Geometry check sheet. Reference: the model listing, model coordinates, mm. Round coordinates to 2 decimals unless told otherwise and drop trailing zeros. Loops run counter-clockwise (first coordinate to the right, second up) from the corner with the lowest first, then second, coordinate; pieces in that order, holes last. Notation, with made-up numbers: M -29,-33.5 L -7,-33.5 A21 ccw -7,-20.5 Z; hole C 18.5,55.5 d9. An arc over 180 degrees is marked long. Write item = value, one per line.
from build123d import *

# Parameters (mm, degrees)
F1_DEPTH = 3.048


with BuildPart() as f1:
    # F0 (on Front) → F1 (new body)
    with BuildSketch(Plane.XZ):
        with BuildLine():
            ThreePointArc((6.209856088, 64.9557709646), (6.2206928765, 65.1675907882), (6.224306538, 65.3796568513))
            ThreePointArc((6.224306538, 65.3796568513), (-2.0871396142, 71.2436009258), (-4.824583776, 61.4470517012))
            ThreePointArc((-4.824583776, 61.4470517012), (-2.6706040451, 59.7573916572), (0, 59.1553503133))
            ThreePointArc((0, 59.1553503133), (4.2487407654, 60.8310093834), (6.209856088, 64.9557709646))
        make_face()
        with BuildLine():
            ThreePointArc((0, 59.1553503133), (-2.6706040451, 59.7573916572), (-4.824583776, 61.4470517012))
            Line((-4.824583776, 61.4470517012), (-8.1232850213, 47.4475871287))
            ThreePointArc((-8.1232850213, 47.4475871287), (-5.1805872599, 52.0766598943), (0, 53.8792414952))
            Line((0, 53.8792414952), (0, 59.1553503133))
        make_face()
        with BuildLine():
            Line((7.9024256694, 48.2173679334), (6.209856088, 64.9557709646))
            ThreePointArc((6.209856088, 64.9557709646), (4.2487407654, 60.8310093834), (0, 59.1553503133))
            Line((0, 59.1553503133), (0, 53.8792414952))
            ThreePointArc((0, 53.8792414952), (4.8606878035, 52.3176828203), (7.9024256694, 48.2173679334))
        make_face()
        with BuildLine():
            ThreePointArc((0, 53.8792414952), (-5.1805872599, 52.0766598943), (-8.1232850213, 47.4475871287))
            ThreePointArc((-8.1232850213, 47.4475871287), (-6.5431667331, 40.3529059013), (0, 37.1877448272))
            Line((0, 37.1877448272), (0, 53.8792414952))
        make_face()
        with BuildLine():
            ThreePointArc((0, 37.1877448272), (-6.5431667331, 40.3529059013), (-8.1232850213, 47.4475871287))
            Line((-8.1232850213, 47.4475871287), (-8.9761791751, 43.8279621303))
            Line((-8.9761791751, 43.8279621303), (-7.522948678, 9.569606592))
            Line((-7.522948678, 9.569606592), (-5.7813609054, 9.6774364228))
            ThreePointArc((-5.7813609054, 9.6774364228), (-3.1997914593, 11.7007529388), (0, 12.4216171046))
            Line((0, 12.4216171046), (0, 37.1877448272))
        make_face()
        with BuildLine():
            Line((8.2797434874, 44.4859421904), (7.9024256694, 48.2173679334))
            ThreePointArc((7.9024256694, 48.2173679334), (4.8606878035, 52.3176828203), (0, 53.8792414952))
            Line((0, 53.8792414952), (0, 37.1877448272))
            ThreePointArc((0, 37.1877448272), (5.5185559019, 39.2727379343), (8.2797434874, 44.4859421904))
        make_face()
        with BuildLine():
            ThreePointArc((8.345748334, 45.5334931612), (8.2341718199, 46.893614367), (7.9024256694, 48.2173679334))
            Line((7.9024256694, 48.2173679334), (8.2797434874, 44.4859421904))
            ThreePointArc((8.2797434874, 44.4859421904), (8.3292307769, 45.0086789855), (8.345748334, 45.5334931612))
        make_face()
        with BuildLine():
            ThreePointArc((8.2797434874, 44.4859421904), (5.5185559019, 39.2727379343), (0, 37.1877448272))
            Line((0, 37.1877448272), (0, 12.4216171046))
            ThreePointArc((0, 12.4216171046), (5.2764963843, 10.2360207404), (7.4620927485, 4.9595243561))
            ThreePointArc((7.4620927485, 4.9595243561), (7.4592970858, 4.7552814289), (7.4509121924, 4.5511915405))
            Line((7.4509121924, 4.5511915405), (9.1615496203, 35.7654578984))
            Line((9.1615496203, 35.7654578984), (8.2797434874, 44.4859421904))
        make_face()
        with BuildLine():
            ThreePointArc((7.4620927485, 4.9595243561), (5.2764963843, 10.2360207404), (0, 12.4216171046))
            ThreePointArc((0, 12.4216171046), (-3.1997914593, 11.7007529388), (-5.7813609054, 9.6774364228))
            ThreePointArc((-5.7813609054, 9.6774364228), (-6.8181639984, 7.9919273436), (-7.3754788979, 6.0931641639))
            Line((-7.3754788979, 6.0931641639), (-7.2529785413, 3.2053492032))
            ThreePointArc((-7.2529785413, 3.2053492032), (-6.1468484582, 0.7287936603), (-4.2285927984, -1.1887950186))
            ThreePointArc((-4.2285927984, -1.1887950186), (3.2913062747, -1.737499699), (7.4509121924, 4.5511915405))
            ThreePointArc((7.4509121924, 4.5511915405), (7.4592970858, 4.7552814289), (7.4620927485, 4.9595243561))
        make_face()
        with BuildLine():
            Line((-5.7813609054, 9.6774364228), (-7.522948678, 9.569606592))
            Line((-7.522948678, 9.569606592), (-7.3754788979, 6.0931641639))
            ThreePointArc((-7.3754788979, 6.0931641639), (-6.8181639984, 7.9919273436), (-5.7813609054, 9.6774364228))
        make_face()
        with BuildLine():
            Line((-7.3754788979, 6.0931641639), (-7.522948678, 9.569606592))
            Line((-7.522948678, 9.569606592), (-39.5340041513, 7.5876526823))
            ThreePointArc((-39.5340041513, 7.5876526823), (-38.8517853204, 6.0251107225), (-38.6185603593, 4.3361566003))
            ThreePointArc((-38.6185603593, 4.3361566003), (-38.6444768889, 3.7683918186), (-38.7220109269, 3.2053492032))
            Line((-38.7220109269, 3.2053492032), (-7.2529785413, 3.2053492032))
            ThreePointArc((-7.2529785413, 3.2053492032), (-7.4553880231, 4.6432687427), (-7.3754788979, 6.0931641639))
        make_face()
        with BuildLine():
            ThreePointArc((-38.6185603593, 4.3361566003), (-38.8517853204, 6.0251107225), (-39.5340041513, 7.5876526823))
            ThreePointArc((-39.5340041513, 7.5876526823), (-50.8562066327, 6.0011927176), (-41.9672696546, -1.1887950186))
            ThreePointArc((-41.9672696546, -1.1887950186), (-39.8375427183, 0.6337643909), (-38.7220109269, 3.2053492032))
            ThreePointArc((-38.7220109269, 3.2053492032), (-38.6444768889, 3.7683918186), (-38.6185603593, 4.3361566003))
        make_face()
        with BuildLine():
            ThreePointArc((-4.2285927984, -1.1887950186), (-6.1468484582, 0.7287936603), (-7.2529785413, 3.2053492032))
            Line((-7.2529785413, 3.2053492032), (-38.7220109269, 3.2053492032))
            ThreePointArc((-38.7220109269, 3.2053492032), (-39.8375427183, 0.6337643909), (-41.9672696546, -1.1887950186))
            Line((-41.9672696546, -1.1887950186), (-4.2285927984, -1.1887950186))
        make_face()
    extrude(amount=F1_DEPTH)


solid = f1.part
(1) Release check for a two-part mould opening along X. For faces 1 (the flat face through (-23, -2, -1.189)), 2 (the flat face through (8.727, -1.503, 40.065)), 3 (the flat face through (-8, -3.048, 26)) record: released by +X, released by -X, zero draft, split by the parting line, or undercut.
Result set:
face_1 = undercut
face_2 = released by +X
face_3 = zero draft
(2) Sectioned sample at C-C on z = 15.5. Record the cut outline in (x, y), then the cut area to 3 significant figures.
Result set:
outline = M -7.77,-3.05 L 8.05,-3.05 L 8.05,0 L -7.77,0 Z
area = 48.2 mm2
(3) Sectioned sample at B-B on x = -20. Record the cut outline in (y, z).
Result set:
outline = M -3.05,-1.19 L 0,-1.19 L 0,8.8 L -3.05,8.8 Z
(4) Sectioned sample at A-A on y = -1.8. Record the cut outline in (x, z).
Result set:
outline = M -41.97,-1.19 L -4.23,-1.19 A7.46 ccw 7.45,4.55 L 9.16,35.77 L 8.28,44.49 A8.35 ccw 7.9,48.22 L 6.21,64.96 A6.22 ccw long -4.82,61.45 L -8.98,43.83 L -7.52,9.57 L -39.53,7.59 A6.23 ccw long Z; hole M -7.38,6.09 A7.46 ccw -7.25,3.21 Z
(5) Material ranges on line 1 along Z through (x, y) = (-27, -1.5); line 2 along X through (y, z) = (-1.8, 49); line 3 along Z through (x, y) = (-22, -0.2), recorded low to high. Write a range as from..to.
Result set:
line_1 = -1.19..8.36
line_2 = -7.76..7.82
line_3 = -1.19..8.67
(6) Depth check by flat-ended pin: pin 1 Ø1.5 at (x, y) = (-20.5, -1.5) entering from -Z. Enter the tip coordinate at first touch or a pass-through.
Result set:
pin_1 = -1.19
